Here's how the part is built. I have some questions about the finished solid (model axes, mm). A direction names the side the tool comes from. Round coordinates to 2 decimals unless told otherwise and drop trailing zeros. Loops run counter-clockwise (first coordinate to the right, second up) from the corner with the lowest first, then second, coordinate; pieces in that order, holes last. Notation, with made-up numbers: M 29,-24.5 L 39,-24.5 A15 ccw 39,3.5 Z; hole C -23,86.25 d8. An arc over 180 degrees is marked long. Use a Markdown table: item, result.
```python
from build123d import *

# Parameters (mm, degrees)
SKETCH1_W           = 41.91
SKETCH1_H           = 4.3561
BOSS_EXTRUDE1_DEPTH = 3.429
CUT_EXTRUDE1_DEPTH  = 3.429
CUT_EXTRUDE2_START  = -3.429
CUT_EXTRUDE2_DEPTH  = 3.429


with BuildPart() as part:
    # Sketch1 → Boss-Extrude1 (new body)
    with BuildSketch(Plane(origin=(0, 0, 0), x_dir=(1, 0, 0), z_dir=(0, 1, 0))):
        with Locations((20.955, 2.17805)):
            Rectangle(SKETCH1_W, SKETCH1_H)
    extrude(amount=BOSS_EXTRUDE1_DEPTH)

    # Sketch3 → Cut-Extrude1 (cut)
    with BuildSketch(Plane(origin=(0, 3.429, 0), x_dir=(1, 0, 0), z_dir=(0, 1, 0))):
        with BuildLine():
            Line((3.2131, 0), (3.2131, 0.673406365))
            ThreePointArc((3.2131, 0.673406365), (3.810306846, 1.27), (4.406900482, 0.672793154))
            Line((4.406900482, 0.672793154), (4.406900482, 0))
            Line((4.406900482, 0), (3.2131, 0))
        make_face()
        with BuildLine():
            Line((9.918700482, 0), (9.918700482, 0.7112))
            ThreePointArc((9.918700482, 0.7112), (10.477500482, 1.27), (11.036300482, 0.7112))
            Line((11.036300482, 0.7112), (11.036300482, 0))
            Line((11.036300482, 0), (9.918700482, 0))
        make_face()
        with BuildLine():
            Line((16.624300482, 0), (16.624300482, 0.7493))
            ThreePointArc((16.624300482, 0.7493), (17.145000482, 1.27), (17.665700482, 0.7493))
            Line((17.665700482, 0.7493), (17.665700482, 0))
            Line((17.665700482, 0), (16.624300482, 0))
        make_face()
        with BuildLine():
            Line((23.304500482, 0), (23.304500482, 0.8509))
            ThreePointArc((23.304500482, 0.8509), (23.723600482, 1.27), (24.142700482, 0.8509))
            Line((24.142700482, 0.8509), (24.142700482, 0))
            Line((24.142700482, 0), (23.304500482, 0))
        make_face()
        with BuildLine():
            Line((29.781500482, 0), (29.781500482, 0.9144))
            ThreePointArc((29.781500482, 0.9144), (30.137100482, 1.27), (30.492700482, 0.9144))
            Line((30.492700482, 0.9144), (30.492700482, 0))
            Line((30.492700482, 0), (29.781500482, 0))
        make_face()
        with BuildLine():
            Line((36.537900482, 0), (36.537900482, 0.9525))
            ThreePointArc((36.537900482, 0.9525), (36.855400482, 1.27), (37.172900482, 0.9525))
            Line((37.172900482, 0.9525), (37.172900482, 0))
            Line((37.172900482, 0), (36.537900482, 0))
        make_face()
    extrude(amount=-CUT_EXTRUDE1_DEPTH, mode=Mode.SUBTRACT)

    # Sketch4 → Cut-Extrude2 (cut)
    with BuildSketch(Plane(origin=(0, 3.429, 0), x_dir=(1, 0, 0), z_dir=(0, 1, 0)).offset(CUT_EXTRUDE2_START)):
        with BuildLine():
            Line((0, 0.508), (0, -0.53864271))
            Line((0, -0.53864271), (41.91, -0.53864271))
            Line((41.91, -0.53864271), (41.91, 0.508))
            ThreePointArc((41.91, 0.508), (20.955, 0), (0, 0.508))
        make_face()
    extrude(amount=CUT_EXTRUDE2_DEPTH, mode=Mode.SUBTRACT)


solid = part.part
```
Q1. I need wall thicknesses on line 1 (Z direction, x = 23, y = 1.5); line 2 (Z direction, x = 31, y = 1.7). Which ranges of each line are inside material? Lowest first, please. Write a range as from..to.
Return value:
| item | result |
|---|---|
| line 1 | z = -4.36..0 |
| line 2 | z = -4.36..-0.12 |
Q2. For faces 4 (the flat face through (21, 3.429, -2)), 5 (the flat face through (29.782, 1.7, -0.5)), 6 (the cylindrical face through (27.002, 1.69, -0.042)), 7 (the cylindrical face through (13.87, 1.69, -0.06)), which set-ups out of +Z, -Z, +X, -X, +Y, -Y let a thin tool reach every point of the face, with its end or its side?
Return value:
| item | result |
|---|---|
| face 4 | +Z, -Z, +X, -X, +Y |
| face 5 | +Z, +Y, -Y |
| face 6 | +Z, +X, +Y, -Y |
| face 7 | +Z, -X, +Y, -Y |
Q3. Imagine slicing it at C-C, the plane x = 29. Please give me the cut outline in (y, z).
Return value:
| item | result |
|---|---|
| outline | M 0,-4.36 L 3.43,-4.36 L 3.43,-0.07 L 0,-0.07 Z |
Q4. We'd pull the mould along X, two halves only. Please class faces 1 (the flat face through (24.143, 1.7, -0.4)), 2 (the flat face through (21, 0, -2)), 3 (the cylindrical face through (39.57, 1.69, -0.4)): pulls with the +X half, pulls with the -X half, needs draft (parallel to the pull), parting line crosses it, or undercut.
Return value:
| item | result |
|---|---|
| face 1 | undercut |
| face 2 | needs draft |
| face 3 | pulls with the +X half |
Q5. Imagine slicing it at B-B, the plane x = 3.81. Please give me the cut outline in (y, z), then the cut area to 3 significant figures.
Return value:
| item | result |
|---|---|
| outline | M 0,-4.36 L 3.43,-4.36 L 3.43,-1.27 L 0,-1.27 Z |
| area | 10.6 mm^2 |
